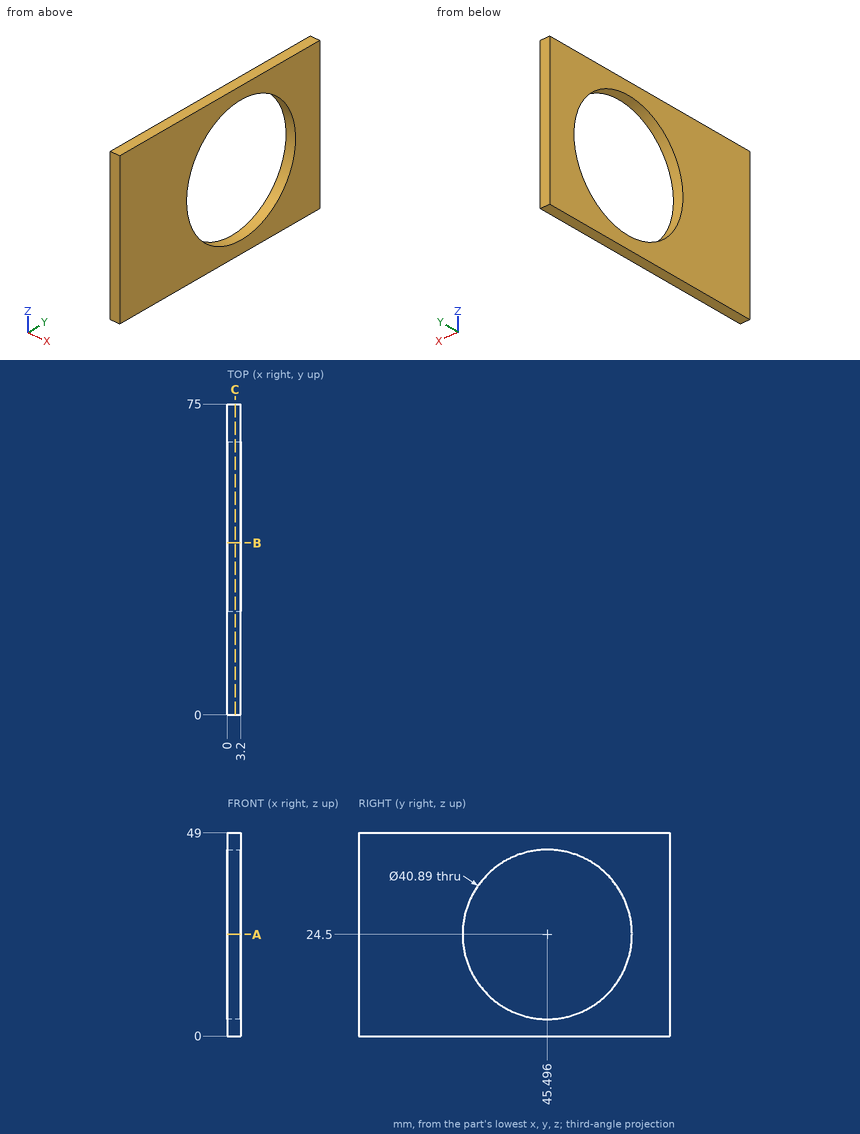
Geometry: see drawing. Coordinates: mm, zero at the bounding-box minimum. Give positions to 0.01 mm unless a question says otherwise; leave off trailing zeros. Write each loop counter-clockwise with the first axis right and the second up, starting at its lowest first coordinate (ties: lowest second). Pieces come first, ordered by that corner, then holes. Notation, with made-up numbers: M 59.5,22.25 L 117.5,22.25 A30 cw 117.5,49.25 Z; hole C -0.5,-35.75 d5. An arc over 180 degrees is marked long. Return JSON: item names as keys, results as strings. Group by question number.
1) Ray query, L1, parallel to Y at x = 1.8, z = 24.5; L2, parallel to Z at x = 0.6, y = 45; L3, parallel to Z at x = 3.1, y = 61. Return the intervals inside material, ascending.
2) Cut plane B-B, the plane y = 41.5. Output: boundary loops of the cut face in (x, z), then the cut area to 3 significant figures.
3) Cut plane C-C, the plane x = 1.85. Output: boundary loops of the cut face in (y, z) (1 decimal), then the cut area to 3 significant figures.
4) First-contact query: pin 1 Ø2 at (y, z) = (43, 6.5) entering from -X. Flat tip, straight axial feed; report the tip coordinate or a pass-through.
5) Cut plane A-A, the plane z = 24.5. Output: boundary loops of the cut face in (x, y).
Data:
{
 "1": {"L1": "y = 0 to 25.05, 65.94 to 75", "L2": "z = 0 to 4.06, 44.94 to 49", "L3": "z = 0 to 11.17, 37.83 to 49"},
 "2": {"outline": "M 0,0 L 3.2,0 L 3.2,4.45 L 0,4.45 Z; M 0,44.55 L 3.2,44.55 L 3.2,49 L 0,49 Z", "area": "28.5 mm²"},
 "3": {"outline": "M 0,0 L 75,0 L 75,49 L 0,49 Z; hole C 45.5,24.5 d40.9", "area": "2,360 mm²"},
 "4": {"pin 1": "passes through"},
 "5": {"outline": "M 0,0 L 3.2,0 L 3.2,25.05 L 0,25.05 Z; M 0,65.94 L 3.2,65.94 L 3.2,75 L 0,75 Z"}
}
